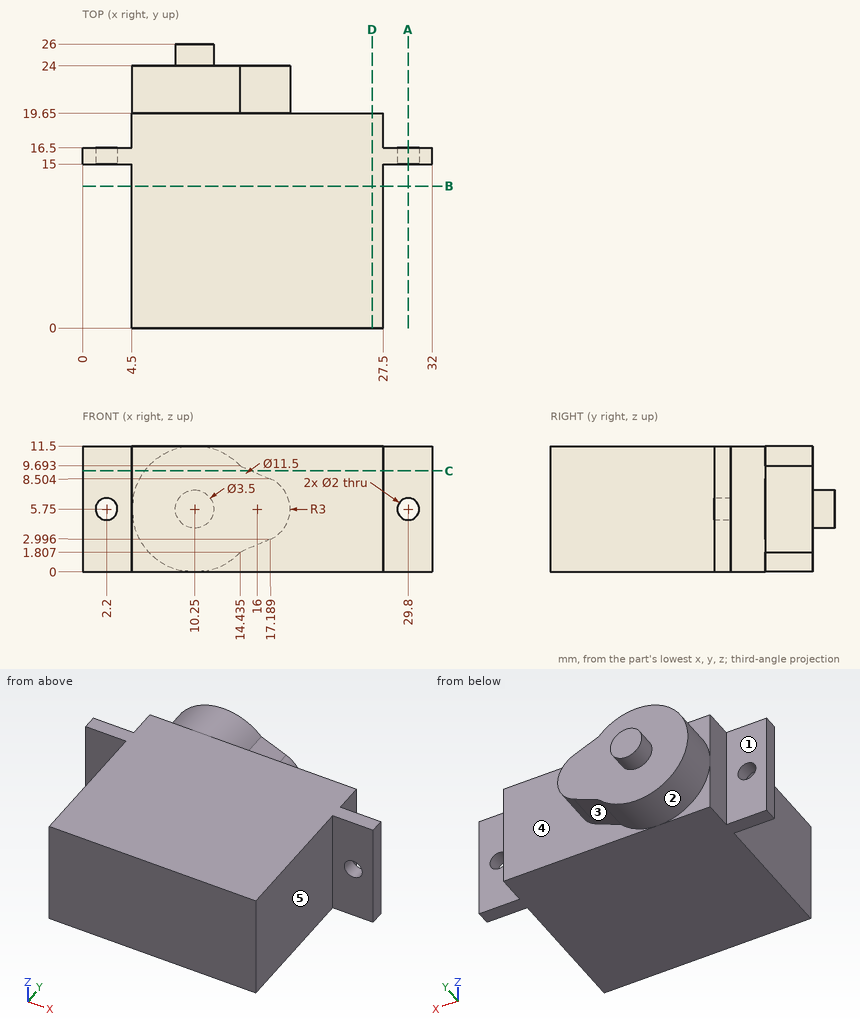
The figure shows three views and two pictorial views of one solid part (mm, origin at its lowest corner). Answer the questions. A direction names the side the tool comes from. Coordinates: 2 decimals unless noted, no trailing zeros. Order: outer loops, then holes, each group sorted by start corner. A loop starts at its lowest first (then second) coordinate and runs counter-clockwise, first axis right, second up. Notation, with made-up numbers: (3, -31.5) - (48, -31.5) arc R19 cw to (48, 5.5) - close; hole circle Ø1 at (26, 40). An arc over 180 degrees is marked (long way). Answer as a JSON object with one key per item and string values.
1. A tool of negligible diameter and unlimited length cuts with its end or side. For the marked faces 1, 2, 3, 4 and 5, from which of +Z, -Z, +X, -X, +Y, -Y can it reach the whole face along a straight path? Write none if from no direction.
Output values:
{"face 1": "+Z, -Z, -X, +Y", "face 2": "+Y", "face 3": "-Z, +X, +Y", "face 4": "+X, +Y", "face 5": "+Z, -Z, +X, -Y"}
2. Consider line 1 (X direction, y = 16.1, z = 5.75); line 2 (Y direction, x = 19.5, z = 3.75); line 3 (X direction, y = 4.75, z = 9.5). Determine where each line is inside the solid, lowest interval first.
Output values:
{"line 1": "x = 0 to 1.2, 3.2 to 28.8, 30.8 to 32", "line 2": "y = 0 to 19.65", "line 3": "x = 4.5 to 27.5"}
3. Find section B-B on y = 13. Determine the outline of the cut face in (x, z).
Output values:
{"outline": "(4.5, 0) - (27.5, 0) - (27.5, 11.5) - (4.5, 11.5) - close"}
4. Each of these flat-tipped pins is pushed along its axis until it touches: P1, Ø5, axis at x = 3, z = 3, coming from the +Y side; P2, Ø3, axis at x = 29.8, z = 5.75, coming from the -Y side; P3, Ø2.5, axis at x = 2.2, z = 5.75, coming from the +Y side. Where does it stop, or does it pass through?
Output values:
{"P1": "stops at y = 24", "P2": "stops at y = 15", "P3": "stops at y = 16.5"}
5. Find section C-C on z = 9.25. Determine the outline of the cut face in (x, y), plus the area to 3 significant figures.
Output values:
{"outline": "(0, 15) - (4.5, 15) - (4.5, 0) - (27.5, 0) - (27.5, 15) - (32, 15) - (32, 16.5) - (27.5, 16.5) - (27.5, 19.65) - (15.46, 19.65) - (15.46, 24) - (5.69, 24) - (5.69, 19.65) - (4.5, 19.65) - (4.5, 16.5) - (0, 16.5) - close", "area": "508 mm²"}
6. Find section D-D on x = 26.5. Determine the outline of the cut face in (y, z).
Output values:
{"outline": "(0, 0) - (19.65, 0) - (19.65, 11.5) - (0, 11.5) - close"}
7. Find section A-A on x = 29.8. Determine the outline of the cut face in (y, z).
Output values:
{"outline": "(15, 0) - (16.5, 0) - (16.5, 4.75) - (15, 4.75) - close; (15, 6.75) - (16.5, 6.75) - (16.5, 11.5) - (15, 11.5) - close"}
